Read the model definition and answer for the solid it produces. Units are mm, in the model's axes. A direction names the side the tool comes from. Give positions to 0.01 mm unless a question says otherwise; leave off trailing zeros. Order: outer loops, then holes, each group sorted by start corner. A loop starts at its lowest first (then second) coordinate and runs counter-clockwise, first axis right, second up. Notation, with made-up numbers: (-27, 27) -> (-16, 27) arc R17 cw to (-16, 46) -> close; hole circle Ø2 at (0.25, 30.25). An arc over 180 degrees is marked (long way). Use one line per item in the form item = value.
```python
from build123d import *

# Parameters (mm, degrees)
BOSS_EXTRUDE8_DEPTH  = 4
BOSS_EXTRUDE10_DEPTH = 8
BOSS_EXTRUDE11_DEPTH = 4


with BuildPart() as part:
    # Sketch11 → Boss-Extrude8 (new body)
    with BuildSketch(Plane(origin=(0, 0, 0), x_dir=(1, 0, 0), z_dir=(0, 1, 0))):
        with BuildLine():
            Line((27.930717857, -16.617009358), (41.012193309, -29.69848481))
            Line((41.012193309, -29.69848481), (43.08274567, -37.42589142))
            Line((43.08274567, -37.42589142), (37.42589142, -43.08274567))
            Line((37.42589142, -43.08274567), (29.69848481, -41.012193309))
            Line((29.69848481, -41.012193309), (16.617009358, -27.930717857))
            ThreePointArc((16.617009358, -27.930717857), (0, -32.5), (-16.617009358, -27.930717857))
            Line((-16.617009358, -27.930717857), (-29.69848481, -41.012193309))
            Line((-29.69848481, -41.012193309), (-37.42589142, -43.08274567))
            Line((-37.42589142, -43.08274567), (-43.08274567, -37.42589142))
            Line((-43.08274567, -37.42589142), (-41.012193309, -29.69848481))
            Line((-41.012193309, -29.69848481), (-27.930717857, -16.617009358))
            ThreePointArc((-27.930717857, -16.617009358), (-32.5, 0), (-27.930717857, 16.617009358))
            Line((-27.930717857, 16.617009358), (-41.012193309, 29.69848481))
            Line((-41.012193309, 29.69848481), (-43.08274567, 37.42589142))
            Line((-43.08274567, 37.42589142), (-37.42589142, 43.08274567))
            Line((-37.42589142, 43.08274567), (-29.69848481, 41.012193309))
            Line((-29.69848481, 41.012193309), (-16.617009358, 27.930717857))
            ThreePointArc((-16.617009358, 27.930717857), (0, 32.5), (16.617009358, 27.930717857))
            Line((16.617009358, 27.930717857), (29.69848481, 41.012193309))
            Line((29.69848481, 41.012193309), (37.42589142, 43.08274567))
            Line((37.42589142, 43.08274567), (43.08274567, 37.42589142))
            Line((43.08274567, 37.42589142), (41.012193309, 29.69848481))
            Line((41.012193309, 29.69848481), (27.930717857, 16.617009358))
            ThreePointArc((27.930717857, 16.617009358), (32.5, 0), (27.930717857, -16.617009358))
        make_face()
    extrude(amount=BOSS_EXTRUDE8_DEPTH)

    # Sketch12 → Boss-Extrude10 (add)
    with BuildSketch(Plane(origin=(0, 4, 0), x_dir=(1, 0, 0), z_dir=(0, 1, 0))):
        with BuildLine():
            Line((38.890872967, 31.819805152), (41.012193309, 29.69848481))
            Line((41.012193309, 29.69848481), (26.10190255, 14.788194051))
            ThreePointArc((26.10190255, 14.788194051), (27.250407583, 12.546524879), (28.206823147, 10.216414633))
            Line((28.206823147, 10.216414633), (30.585684682, 10.9893536))
            ThreePointArc((30.585684682, 10.9893536), (30.90933678, 10.043052317), (31.203718671, 9.087240568))
            Line((31.203718671, 9.087240568), (28.824857136, 8.3143016))
            ThreePointArc((28.824857136, 8.3143016), (29.630650218, 4.693033951), (29.983328701, 1))
            Line((29.983328701, 1), (32.484611742, 1))
            ThreePointArc((32.484611742, 1), (32.5, 0), (32.484611742, -1))
            Line((32.484611742, -1), (29.983328701, -1))
            ThreePointArc((29.983328701, -1), (29.630650218, -4.693033951), (28.824857136, -8.3143016))
            Line((28.824857136, -8.3143016), (31.203718671, -9.087240568))
            ThreePointArc((31.203718671, -9.087240568), (30.90933678, -10.043052317), (30.585684682, -10.9893536))
            Line((30.585684682, -10.9893536), (28.206823147, -10.216414633))
            ThreePointArc((28.206823147, -10.216414633), (27.250407583, -12.546524879), (26.10190255, -14.788194051))
            Line((26.10190255, -14.788194051), (41.012193309, -29.69848481))
            Line((41.012193309, -29.69848481), (38.890872965, -31.819805153))
            ThreePointArc((38.890872965, -31.819805153), (38.890872965, -38.890872967), (31.819805152, -38.890872967))
            Line((31.819805152, -38.890872967), (29.69848481, -41.012193309))
            Line((29.69848481, -41.012193309), (14.788194051, -26.10190255))
            ThreePointArc((14.788194051, -26.10190255), (12.546524879, -27.250407583), (10.216414633, -28.206823147))
            Line((10.216414633, -28.206823147), (10.9893536, -30.585684682))
            ThreePointArc((10.9893536, -30.585684682), (10.043052317, -30.90933678), (9.087240568, -31.203718671))
            Line((9.087240568, -31.203718671), (8.3143016, -28.824857136))
            ThreePointArc((8.3143016, -28.824857136), (4.693033951, -29.630650218), (1, -29.983328701))
            Line((1, -29.983328701), (1, -32.484611742))
            ThreePointArc((1, -32.484611742), (0, -32.5), (-1, -32.484611742))
            Line((-1, -32.484611742), (-1, -29.983328701))
            ThreePointArc((-1, -29.983328701), (-4.693033951, -29.630650218), (-8.3143016, -28.824857136))
            Line((-8.3143016, -28.824857136), (-9.087240568, -31.203718671))
            ThreePointArc((-9.087240568, -31.203718671), (-10.043052317, -30.90933678), (-10.9893536, -30.585684682))
            Line((-10.9893536, -30.585684682), (-10.216414633, -28.206823147))
            ThreePointArc((-10.216414633, -28.206823147), (-12.546524879, -27.250407583), (-14.788194051, -26.10190255))
            Line((-14.788194051, -26.10190255), (-29.69848481, -41.012193309))
            Line((-29.69848481, -41.012193309), (-31.819805153, -38.890872965))
            ThreePointArc((-31.819805153, -38.890872965), (-38.890872967, -38.890872965), (-38.890872967, -31.819805152))
            Line((-38.890872967, -31.819805152), (-41.012193309, -29.69848481))
            Line((-41.012193309, -29.69848481), (-26.10190255, -14.788194051))
            ThreePointArc((-26.10190255, -14.788194051), (-27.250407583, -12.546524879), (-28.206823147, -10.216414633))
            Line((-28.206823147, -10.216414633), (-30.585684682, -10.9893536))
            ThreePointArc((-30.585684682, -10.9893536), (-30.90933678, -10.043052317), (-31.203718671, -9.087240568))
            Line((-31.203718671, -9.087240568), (-28.824857136, -8.3143016))
            ThreePointArc((-28.824857136, -8.3143016), (-29.630650218, -4.693033951), (-29.983328701, -1))
            Line((-29.983328701, -1), (-32.484611742, -1))
            ThreePointArc((-32.484611742, -1), (-32.5, 0), (-32.484611742, 1))
            Line((-32.484611742, 1), (-29.983328701, 1))
            ThreePointArc((-29.983328701, 1), (-29.630650218, 4.693033951), (-28.824857136, 8.3143016))
            Line((-28.824857136, 8.3143016), (-31.203718671, 9.087240568))
            ThreePointArc((-31.203718671, 9.087240568), (-30.90933678, 10.043052317), (-30.585684682, 10.9893536))
            Line((-30.585684682, 10.9893536), (-28.206823147, 10.216414633))
            ThreePointArc((-28.206823147, 10.216414633), (-27.250407583, 12.546524879), (-26.10190255, 14.788194051))
            Line((-26.10190255, 14.788194051), (-41.012193309, 29.69848481))
            Line((-41.012193309, 29.69848481), (-38.890872965, 31.819805153))
            ThreePointArc((-38.890872965, 31.819805153), (-38.890872965, 38.890872967), (-31.819805152, 38.890872967))
            Line((-31.819805152, 38.890872967), (-29.69848481, 41.012193309))
            Line((-29.69848481, 41.012193309), (-14.788194051, 26.10190255))
            ThreePointArc((-14.788194051, 26.10190255), (-12.546524879, 27.250407583), (-10.216414633, 28.206823147))
            Line((-10.216414633, 28.206823147), (-10.9893536, 30.585684682))
            ThreePointArc((-10.9893536, 30.585684682), (-10.043052317, 30.90933678), (-9.087240568, 31.203718671))
            Line((-9.087240568, 31.203718671), (-8.3143016, 28.824857136))
            ThreePointArc((-8.3143016, 28.824857136), (-4.693033951, 29.630650218), (-1, 29.983328701))
            Line((-1, 29.983328701), (-1, 32.484611742))
            ThreePointArc((-1, 32.484611742), (0, 32.5), (1, 32.484611742))
            Line((1, 32.484611742), (1, 29.983328701))
            ThreePointArc((1, 29.983328701), (4.693033951, 29.630650218), (8.3143016, 28.824857136))
            Line((8.3143016, 28.824857136), (9.087240568, 31.203718671))
            ThreePointArc((9.087240568, 31.203718671), (10.043052317, 30.90933678), (10.9893536, 30.585684682))
            Line((10.9893536, 30.585684682), (10.216414633, 28.206823147))
            ThreePointArc((10.216414633, 28.206823147), (12.546524879, 27.250407583), (14.788194051, 26.10190255))
            Line((14.788194051, 26.10190255), (29.69848481, 41.012193309))
            Line((29.69848481, 41.012193309), (31.819805153, 38.890872965))
            ThreePointArc((31.819805153, 38.890872965), (38.890872967, 38.890872965), (38.890872967, 31.819805152))
        make_face()
    extrude(amount=BOSS_EXTRUDE10_DEPTH)

    # Sketch13 → Boss-Extrude11 (add)
    with BuildSketch(Plane(origin=(0, 12, 0), x_dir=(1, 0, 0), z_dir=(0, 1, 0))):
        with BuildLine():
            Line((27.930717857, -16.617009358), (41.012193309, -29.69848481))
            Line((41.012193309, -29.69848481), (43.08274567, -37.42589142))
            Line((43.08274567, -37.42589142), (37.42589142, -43.08274567))
            Line((37.42589142, -43.08274567), (29.69848481, -41.012193309))
            Line((29.69848481, -41.012193309), (16.617009358, -27.930717857))
            ThreePointArc((16.617009358, -27.930717857), (0, -32.5), (-16.617009358, -27.930717857))
            Line((-16.617009358, -27.930717857), (-29.69848481, -41.012193309))
            Line((-29.69848481, -41.012193309), (-37.42589142, -43.08274567))
            Line((-37.42589142, -43.08274567), (-43.08274567, -37.42589142))
            Line((-43.08274567, -37.42589142), (-41.012193309, -29.69848481))
            Line((-41.012193309, -29.69848481), (-27.930717857, -16.617009358))
            ThreePointArc((-27.930717857, -16.617009358), (-32.5, 0), (-27.930717857, 16.617009358))
            Line((-27.930717857, 16.617009358), (-41.012193309, 29.69848481))
            Line((-41.012193309, 29.69848481), (-43.08274567, 37.42589142))
            Line((-43.08274567, 37.42589142), (-37.42589142, 43.08274567))
            Line((-37.42589142, 43.08274567), (-29.69848481, 41.012193309))
            Line((-29.69848481, 41.012193309), (-16.617009358, 27.930717857))
            ThreePointArc((-16.617009358, 27.930717857), (0, 32.5), (16.617009358, 27.930717857))
            Line((16.617009358, 27.930717857), (29.69848481, 41.012193309))
            Line((29.69848481, 41.012193309), (37.42589142, 43.08274567))
            Line((37.42589142, 43.08274567), (43.08274567, 37.42589142))
            Line((43.08274567, 37.42589142), (41.012193309, 29.69848481))
            Line((41.012193309, 29.69848481), (27.930717857, 16.617009358))
            ThreePointArc((27.930717857, 16.617009358), (32.5, 0), (27.930717857, -16.617009358))
        make_face()
    extrude(amount=BOSS_EXTRUDE11_DEPTH)


solid = part.part
```
Item 1: Given pin 1 Ø1.5 at (x, y) = (21.5, 2.5) entering from -Z; pin 2 Ø3 at (x, y) = (-27.5, 5) entering from -Z; pin 3 Ø1.3 at (y, z) = (10, 30.5) entering from +X, each flat-ended and moving along its own axis, determine where each tip first touches the part or whether it passes through.
Checks:
pin_1 = -33.56
pin_2 = -40.31
pin_3 = 40.86
Item 2: The part is cut by section D-D on x = 22. Give the vertices of the cut face in (y, z).
Checks:
outline = (0, -33.31) -> (16, -33.31) -> (16, 33.31) -> (0, 33.31) -> close
Item 3: Straight lines are drawn through the part: L1, parallel to Z at x = 30.5, y = 7.25; L2, parallel to Y at x = -11.5, z = 29; L3, parallel to X at y = 14.5, z = -12.5. For each, find the intervals that lie inside material, in ascending order. Write a range as from..to.
Checks:
L1 = -40.21..-19.19, -10.96..-8.86, -1..1, 8.86..10.96, 19.19..40.21
L2 = 0..4, 12..16
L3 = -30..30
Item 4: Which of the six approach directions +Z, -Z, +X, -X, +Y, -Y give full straight-line access (tool end or side, diameter ignored) to faces 4 (the flat face through (-42.062, 13.972, 33.616)), 5 (the flat face through (-33.508, 1.972, 42.033)), 6 (the flat face through (31, 8, -1)), 7 (the flat face through (1, 8, -31))?
Checks:
face_4 = -X, +Y, -Y
face_5 = +Z, +Y, -Y
face_6 = +X
face_7 = -Z
Item 5: The part is cut by section A-A on y = 13.5. Give the vertices of the cut face in (x, z), and give its area (3 significant figures).
Checks:
outline = (-43.08, -37.43) -> (-37.43, -43.08) -> (-29.7, -41.01) -> (-16.62, -27.93) arc R32.5 ccw to (16.62, -27.93) -> (29.7, -41.01) -> (37.43, -43.08) -> (43.08, -37.43) -> (41.01, -29.7) -> (27.93, -16.62) arc R32.5 ccw to (27.93, 16.62) -> (41.01, 29.7) -> (43.08, 37.43) -> (37.43, 43.08) -> (29.7, 41.01) -> (16.62, 27.93) arc R32.5 ccw to (-16.62, 27.93) -> (-29.7, 41.01) -> (-37.43, 43.08) -> (-43.08, 37.43) -> (-41.01, 29.7) -> (-27.93, 16.62) arc R32.5 ccw to (-27.93, -16.62) -> (-41.01, -29.7) -> close
area = 4,790 mm²
Item 6: The part is cut by section C-C on z = 6. Give the vertices of the cut face in (x, y).
Checks:
outline = (-31.94, 0) -> (31.94, 0) -> (31.94, 4) -> (29.39, 4) -> (29.39, 12) -> (31.94, 12) -> (31.94, 16) -> (-31.94, 16) -> (-31.94, 12) -> (-29.39, 12) -> (-29.39, 4) -> (-31.94, 4) -> close
Item 7: Determine the mould class of faces 1 (the flat face through (-33.453, 7.888, -22.139)), 2 (the flat face through (-8.695, 7.944, 29.998)), 3 (the flat face through (-22.348, 7.888, -33.661)) for opening direction Z: +Z half, -Z half, draft (parallel to the pull), parting line (faces both ways), or undercut.
Checks:
face_1 = undercut
face_2 = +Z half
face_3 = -Z half
Item 8: The part is cut by section B-B on x = -3. Give the vertices of the cut face in (y, z), and give its area (3 significant figures).
Checks:
outline = (0, -32.36) -> (4, -32.36) -> (4, -29.85) -> (12, -29.85) -> (12, -32.36) -> (16, -32.36) -> (16, 32.36) -> (12, 32.36) -> (12, 29.85) -> (4, 29.85) -> (4, 32.36) -> (0, 32.36) -> close
area = 995 mm²
